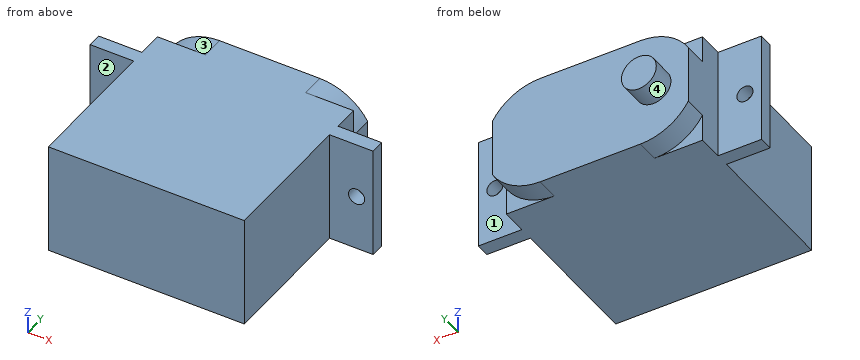
from build123d import *

# Parameters (mm, degrees)
ESQUISSE1_W      = 22.5
ESQUISSE1_H      = 20.5
EXTRUSION1_DEPTH = 12.85
EXTRUSION2_DEPTH = 2.65
ESQUISSE3_W      = 12.85
ESQUISSE3_H      = 1.6
EXTRUSION3_DEPTH = 5
ESQUISSE5_R      = 0.925
EXTRUSION5_DEPTH = 2.75
ESQUISSE4_R      = 2
EXTRUSION4_DEPTH = 2.75


with BuildPart() as part:
    # Esquisse1 → Extrusion1 (new body)
    with BuildSketch(Plane.XY):
        Rectangle(ESQUISSE1_W, ESQUISSE1_H)
    extrude(amount=EXTRUSION1_DEPTH)

    # Esquisse2 → Extrusion2 (add)
    with BuildSketch(Plane(origin=(0, 10.25, 0), x_dir=(1, 0, 0), z_dir=(0, 1, 0))):
        with BuildLine():
            Line((-5.75, 0), (5.75, 0))
            ThreePointArc((5.75, 0), (8.907662728, -0.829484734), (11.25, -3.103761526))
            Line((11.25, -3.103761526), (11.25, -9.746238474))
            ThreePointArc((11.25, -9.746238474), (8.907662728, -12.020515266), (5.75, -12.85))
            Line((5.75, -12.85), (-5.75, -12.85))
            ThreePointArc((-5.75, -12.85), (-8.907662728, -12.020515266), (-11.25, -9.746238474))
            Line((-11.25, -9.746238474), (-11.25, -3.103761526))
            ThreePointArc((-11.25, -3.103761526), (-8.907662728, -0.829484734), (-5.75, 0))
        make_face()
    extrude(amount=EXTRUSION2_DEPTH)

    # Esquisse3 → Extrusion3 (add)
    with BuildSketch(Plane.ZY.offset(11.25)):
        with Locations((6.425, 6.55)):
            Rectangle(ESQUISSE3_W, ESQUISSE3_H)
    extrusion3 = extrude(amount=EXTRUSION3_DEPTH)

    # Esquisse5 → Extrusion5 (cut)
    with BuildSketch(Plane(origin=(0, 7.35, 0), x_dir=(1, 0, 0), z_dir=(0, 1, 0))):
        with Locations(Location((-14.35, -6.425, 0), (0, 0, 270))):
            Circle(ESQUISSE5_R)
    extrusion5 = extrude(amount=-EXTRUSION5_DEPTH, mode=Mode.SUBTRACT)

    # Symétrie1: Extrusion3, Extrusion5 across plane
    add(extrusion3.mirror(Plane(origin=(0, 0, 0), x_dir=(0, 0, 1), z_dir=(1, 0, 0))))
    add(extrusion5.mirror(Plane(origin=(0, 0, 0), x_dir=(0, 0, 1), z_dir=(1, 0, 0))), mode=Mode.SUBTRACT)

    # Esquisse4 → Extrusion4 (add)
    with BuildSketch(Plane(origin=(0, 12.9, 0), x_dir=(1, 0, 0), z_dir=(0, 1, 0))):
        with Locations(Location((-7.25, -6.425, 0), (0, 0, 270))):
            Circle(ESQUISSE4_R)
    extrude(amount=EXTRUSION4_DEPTH)


solid = part.part
Source: CAD feature listing. Evaluate the final solid. Frame: model axes, mm. Face numbers are marked on the shaded views. A direction names the side the tool comes from. Round coordinates to 2 decimals unless told otherwise and drop trailing zeros. Loops run counter-clockwise (first coordinate to the right, second up) from the corner with the lowest first, then second, coordinate; pieces in that order, holes last. Notation, with made-up numbers: (49, 28) - (80, 28) arc R18 cw to (80, 38) - close; hole circle Ø5 at (-22, -12.5). An arc over 180 degrees is marked (long way). Write item = value, one per line. Start each with the question number.
(1) Set-up query: the marked faces 1, 2, 3 and 4. Return all of +Z, -Z, +X, -X, +Y, -Y with unobstructed straight access to the full face (end or side cutting, diameter ignored); none if empty.
(2) Section query A-A, the plane x = -14.35. Output: boundary loops of the cut face in (y, z), plus the area to 3 significant figures.
(3) Pin query (flat end, axial travel): pin 1 (6.5 mm diameter, centred on y = -6, z = 5.5, fed in from +X); pin 2 (3 mm diameter, centred on x = 10.5, z = 2.5, fed in from +Y); pin 3 (1.5 mm diameter, centred on x = -14, z = 6, fed in from +Y); pin 4 (2 mm diameter, centred on x = -10.5, y = 11, fed in from +Z). Return the tip coordinate at first contact, or that it passes through.
(4) Ray query, line 1 along Z through (x, y) = (14.35, 6.4); line 2 along X through (y, z) = (1.5, 2); line 3 along Y through (x, z) = (-4, 9). Return the intervals inside material, ascending. Write a range as from..to.
(5) Section query D-D, the plane y = -1. Output: boundary loops of the cut face in (x, z).
(6) Section query C-C, the plane x = 8.5. Output: boundary loops of the cut face in (y, z).
(7) Section query B-B, the plane z = 6.5. Output: boundary loops of the cut face in (x, y).
Conclusion:
q1.face_1 = +Z, -Z, +X, +Y
q1.face_2 = +Z, -Z, -X, -Y
q1.face_3 = +Z, -X, +Y
q1.face_4 = +Y
q2.outline = (5.75, 0) - (7.35, 0) - (7.35, 5.5) - (5.75, 5.5) - close; (5.75, 7.35) - (7.35, 7.35) - (7.35, 12.85) - (5.75, 12.85) - close
q2.area = 17.6 mm2
q3.pin_1 = 11.25
q3.pin_2 = 12.9
q3.pin_3 = 7.35
q3.pin_4 = 12.85
q4.line_1 = 0..5.5, 7.35..12.85
q4.line_2 = -11.25..11.25
q4.line_3 = -10.25..12.9
q5.outline = (-11.25, 0) - (11.25, 0) - (11.25, 12.85) - (-11.25, 12.85) - close
q6.outline = (-10.25, 0) - (10.25, 0) - (10.25, 0.62) - (12.9, 0.62) - (12.9, 12.23) - (10.25, 12.23) - (10.25, 12.85) - (-10.25, 12.85) - close
q7.outline = (-16.25, 5.75) - (-15.27, 5.75) - (-15.27, 7.35) - (-16.25, 7.35) - close; (-13.43, 5.75) - (-11.25, 5.75) - (-11.25, -10.25) - (11.25, -10.25) - (11.25, 5.75) - (13.43, 5.75) - (13.43, 7.35) - (11.25, 7.35) - (11.25, 12.9) - (-5.25, 12.9) - (-5.25, 15.65) - (-9.25, 15.65) - (-9.25, 12.9) - (-11.25, 12.9) - (-11.25, 7.35) - (-13.43, 7.35) - close; (15.27, 5.75) - (16.25, 5.75) - (16.25, 7.35) - (15.27, 7.35) - close
